Source: three-view drawing plus pictorial views. Frame: mm from the lowest corner of the part. A direction names the side the tool comes from. Give positions to 0.01 mm unless a question says otherwise; leave off trailing zeros. One line per item, written item: value.
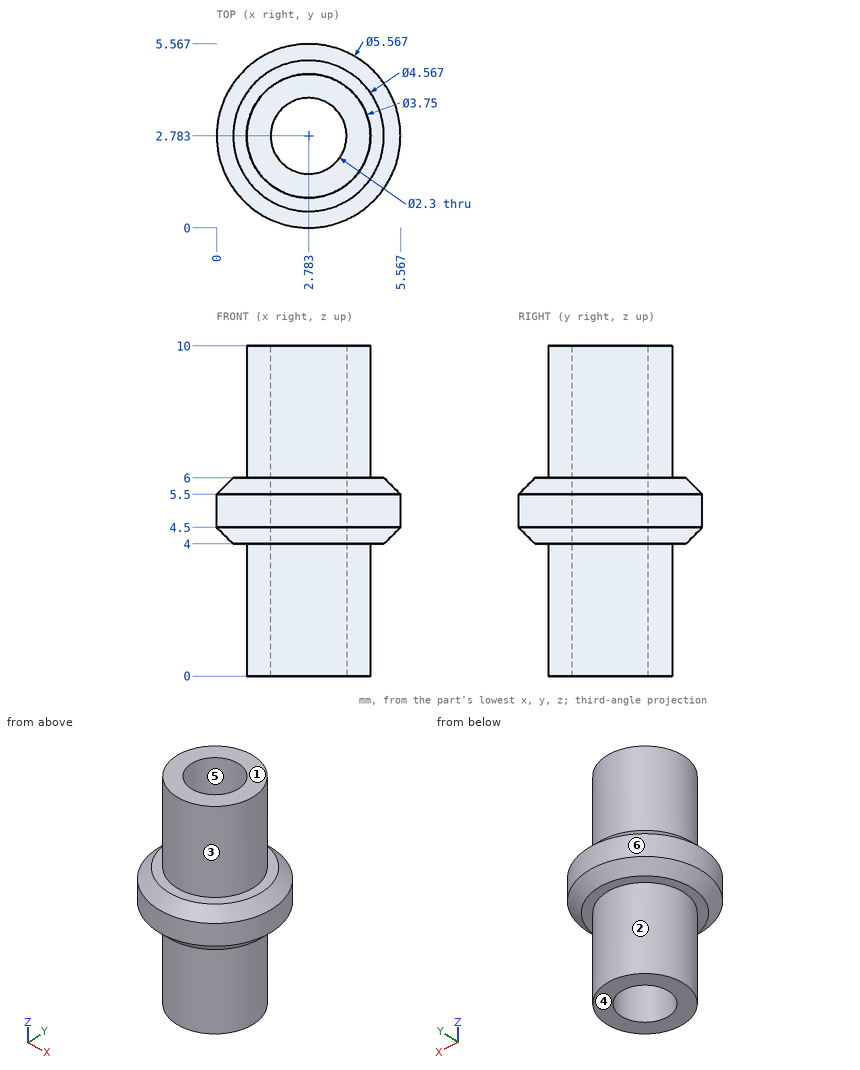
Item 1: Draft query along Y for the marked faces 4, 5 and 6. Return one class per face: pulls with the +Y half, pulls with the -Y half, needs draft (parallel to the pull), parting line crosses it, or undercut.
Verdict:
face 4: needs draft
face 5: undercut
face 6: parting line crosses it
Item 2: Pin query (flat end, axial travel): P1, Ø1.5, axis at x = 4.5, z = 1.5, coming from the +Y side; P2, Ø2, axis at x = 3, z = 8.5, coming from the -Y side. Return the tip coordinate at first contact, or that it passes through.
Verdict:
P1: stops at y = 4.39
P2: stops at y = 0.91
Item 3: Access query for the marked faces 1, 2 and 3. Directions: +Z, -Z, +X, -X, +Y, -Y. A direction counts if a zero-diameter tool reaches every point of the face in a straight line with its end or side. Return the directions, or none.
Verdict:
face 1: +Z, +X, -X, +Y, -Y
face 2: -Z
face 3: +Z
Item 4: Material intervals for L1, parallel to X at y = 3.1, z = 0.5 (1 decimal); L2, parallel to Y at x = 2, z = 6.75 (1 decimal), sorted ascending.
Verdict:
L1: x = 0.9 to 1.7, 3.9 to 4.6
L2: y = 1.1 to 1.9, 3.6 to 4.5
